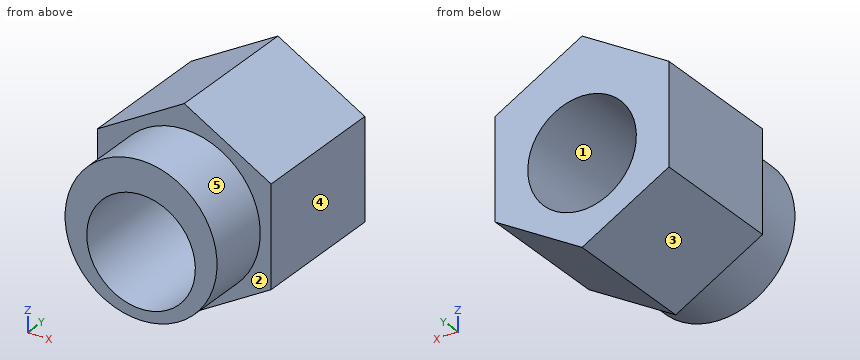
from build123d import *

# Parameters (mm, degrees)
EXTRUDE_1_DEPTH     = 6.5
SKETCH_2_R          = 3.5
SKETCH_2_R_2        = 2.5
EXTRUDE_2_DEPTH     = 3
SKETCH_2_2_R        = 2.5
CUT_EXTRUDE_1_DEPTH = 9.920949127


with BuildPart() as part:
    # Sketch 1 → Extrude 1 (new body)
    with BuildSketch(Plane(origin=(0, 0, 0), x_dir=(1, 0, 0), z_dir=(0, 1, 0))):
        Polygon((0, -4.618802154), (4, -2.309401077), (4, 2.309401077), (0, 4.618802154), (-4, 2.309401077), (-4, -2.309401077), align=None)
    extrude(amount=EXTRUDE_1_DEPTH)

    # Sketch 2 → Extrude 2 (add)
    with BuildSketch(Plane(origin=(0, 0, 0), x_dir=(1, 0, 0), z_dir=(0, 1, 0))):
        with Locations(Location((0, 0, 0), (0, 0, 270))):
            Circle(SKETCH_2_R)
        with Locations(Location((0, 0.5, 0), (0, 0, 270))):
            Circle(SKETCH_2_R_2, mode=Mode.SUBTRACT)
    extrude(amount=-EXTRUDE_2_DEPTH)

    # Sketch 2_2 → Cut-Extrude 1 (cut, through all)
    with BuildSketch(Plane(origin=(0, 0, 0), x_dir=(1, 0, 0), z_dir=(0, 1, 0))):
        with Locations(Location((0, 0.5, 0), (0, 0, 270))):
            Circle(SKETCH_2_2_R)
    extrude(amount=CUT_EXTRUDE_1_DEPTH, mode=Mode.SUBTRACT)


solid = part.part
Geometry: final body of the model. Coordinates: model frame, mm. Face numbers are marked on the shaded views. A direction names the side the tool comes from. Give positions to 0.01 mm unless a question says otherwise; leave off trailing zeros. Order: outer loops, then holes, each group sorted by start corner. A loop starts at its lowest first (then second) coordinate and runs counter-clockwise, first axis right, second up. Notation, with made-up numbers: (67.25, 52.25) - (104.25, 52.25) arc R13 cw to (104.25, 58.25) - close; hole circle Ø9 at (-1.75, 60.5). An arc over 180 degrees is marked (long way). Use CSV: the item, a comma, the result in double quotes.
1. Section query D-D (x = 3). Output: boundary loops of the cut face in (y, z).
Answers below:
outline,"(-3, -1.8) - (0, -1.8) - (0, -2.89) - (6.5, -2.89) - (6.5, 2.89) - (0, 2.89) - (0, 1.8) - (-3, 1.8) - close"
2. Section query C-C (x = 1.5). Output: boundary loops of the cut face in (y, z), plus the area to 3 significant figures.
Answers below:
outline,"(-3, -3.16) - (0, -3.16) - (0, -3.75) - (6.5, -3.75) - (6.5, -2.5) - (-3, -2.5) - close; (-3, 1.5) - (6.5, 1.5) - (6.5, 3.75) - (0, 3.75) - (0, 3.16) - (-3, 3.16) - close"
area,"29.8 mm2"
3. Section query B-B (z = 0). Output: boundary loops of the cut face in (x, y), plus the area to 3 significant figures.
Answers below:
outline,"(-4, 0) - (-3.5, 0) - (-3.5, -3) - (-2.45, -3) - (-2.45, 6.5) - (-4, 6.5) - close; (2.45, -3) - (3.5, -3) - (3.5, 0) - (4, 0) - (4, 6.5) - (2.45, 6.5) - close"
area,"26.5 mm2"
4. Access query for the marked faces 4 and 5. Directions: +Z, -Z, +X, -X, +Y, -Y. A direction counts if a zero-diameter tool reaches every point of the face in a straight line with its end or side. Return the directions, or none.
Answers below:
face 4,"+Z, -Z, +X, +Y, -Y"
face 5,"-Y"
5. Section query A-A (y = 3). Output: boundary loops of the cut face in (x, z), plus the area to 3 significant figures.
Answers below:
outline,"(-4, -2.31) - (0, -4.62) - (4, -2.31) - (4, 2.31) - (0, 4.62) - (-4, 2.31) - close; hole circle Ø5 at (0, -0.5)"
area,"35.8 mm2"
6. Mould query, pull axis Z, two halves, no side actions, for the marked faces 1, 2 and 3. Classes: +Z half, -Z half, draft (parallel to the pull), parting line (faces both ways), or undercut.
Answers below:
face 1,"undercut"
face 2,"draft"
face 3,"-Z half"
7. Material intervals for line 1 along X through (y, z) = (0.75, -0.5); line 2 along Y through (x, z) = (1, -4); line 3 along Z through (x, y) = (1.75, 3.25), sorted ascending. Write a range as from..to.
Answers below:
line 1,"-4..-2.5, 2.5..4"
line 2,"0..6.5"
line 3,"-3.61..-2.29, 1.29..3.61"
